from build123d import *

# Parameters (mm, degrees)
BOSS_EXTRUDE2_DEPTH = 27
BOSS_EXTRUDE3_DEPTH = 27
SKETCH2_W           = 35
SKETCH2_H           = 30
CUT_EXTRUDE1_DEPTH  = 5
FILLET1_R           = 1
SKETCH3_R           = 7.5
CUT_EXTRUDE2_DEPTH  = 1
FILLET2_R           = 1
FILLET3_R           = 1


with BuildPart() as part:
    # Sketch1 → Boss-Extrude2 (new body)
    with BuildSketch(Plane.XY):
        with BuildLine():
            Line((0, -6.138464618), (0, 24))
            Line((0, 24), (-18.5, 24))
            ThreePointArc((-18.5, 24), (-19.98907726, 20.440025069), (-23.569368605, 19.000481223))
            add(Edge.make_bspline(
                [(-38.977266034, 10), (-31.868069792, 12.073515571), (-23.569368605, 19.000481223)],
                knots=[0, 0, 0, 1, 1, 1], degree=2))
            add(Edge.make_bspline(
                [(-42.5, 0), (-60.990919768, 5.63165305), (-38.977266034, 10)],
                knots=[0, 0, 0, 1, 1, 1], degree=2))
            add(Edge.make_bspline(
                [(0, -6.138464618), (-21.18379083, -6.119278693), (-42.5, 0)],
                knots=[0.501567662, 0.501567662, 0.501567662, 1, 1, 1], degree=2))
        make_face()
    extrude(amount=BOSS_EXTRUDE2_DEPTH)

    # Sketch1_4 → Boss-Extrude3 (add)
    with BuildSketch(Plane.XY):
        with BuildLine():
            Line((18.5, 24), (0, 24))
            Line((0, 24), (0, -6.138464618))
            add(Edge.make_bspline(
                [(42.5, 0), (21.317044751, -6.157771231), (0, -6.138464618)],
                knots=[0, 0, 0, 0.501567662, 0.501567662, 0.501567662], degree=2))
            add(Edge.make_bspline(
                [(42.5, 0), (60.990919768, 5.63165305), (38.977266034, 10)],
                knots=[0, 0, 0, 1, 1, 1], degree=2))
            add(Edge.make_bspline(
                [(38.977266034, 10), (31.868069792, 12.073515571), (23.569368605, 19.000481223)],
                knots=[0, 0, 0, 1, 1, 1], degree=2))
            ThreePointArc((23.569368605, 19.000481223), (19.98907726, 20.440025069), (18.5, 24))
        make_face()
    extrude(amount=BOSS_EXTRUDE3_DEPTH)

    # Sketch2 → Cut-Extrude1 (cut)
    with BuildSketch(Plane(origin=(0, 0, 0), x_dir=(-1, 0, 0), z_dir=(0, 0, -1))):
        with Locations((0, 5)):
            Rectangle(SKETCH2_W, SKETCH2_H)
    extrude(amount=-CUT_EXTRUDE1_DEPTH, mode=Mode.SUBTRACT)

    # Fillet1
    fillet1_edges = [part.edges().sort_by_distance(p)[0] for p in [
        (17.5, 20, 2.5),
        (-17.5, 20, 2.5),
    ]]
    fillet(fillet1_edges, radius=FILLET1_R)

    # Sketch3 → Cut-Extrude2 (cut)
    with BuildSketch(Plane(origin=(0, 24, 0), x_dir=(1, 0, 0), z_dir=(0, 1, 0))):
        with Locations(Location((0, -13.5, 0), (0, 0, 270))):
            Circle(SKETCH3_R)
    extrude(amount=-CUT_EXTRUDE2_DEPTH, mode=Mode.SUBTRACT)

    # Fillet2
    fillet2_edges = [part.edges().sort_by_distance(p)[0] for p in [
        (-18.5, 24, 13.5),
    ]]
    fillet(fillet2_edges, radius=FILLET2_R)

    # Fillet3
    fillet3_edges = [part.edges().sort_by_distance(p)[0] for p in [
        (18.5, 24, 13.5),
    ]]
    fillet(fillet3_edges, radius=FILLET3_R)


solid = part.part
Verification items for the finished model (mm, model axes). A direction names the side the tool comes from. Round coordinates to 2 decimals unless told otherwise and drop trailing zeros. Write each loop counter-clockwise with the first axis right and the second up, starting at its lowest first coordinate (ties: lowest second). Pieces come first, ordered by that corner, then holes.
(1) Material ranges on line 1 (X direction, y = 4, z = 1.5); line 2 (X direction, y = 23.2, z = 13.5); line 3 (Z direction, x = 7.5, y = 8), recorded low to high.
Returned:
line 1: x = -50.64 to -17.5, 17.5 to 50.64
line 2: x = -18.56 to -7.5, 7.5 to 18.56
line 3: z = 5 to 27
(2) Access from +Z, -Z, +X, -X, +Y, -Y to the whole of each face (thin tool, end or side, straight path). Record for faces 1 (the cylindrical face through (6.324, 23.507, 17.532)), 2 (the flat face through (-1, 9, 27)), 3 (the flat face through (0, 7, 5)).
Returned:
face 1: +Y
face 2: +Z, +X, -X, +Y, -Y
face 3: -Z, -Y
(3) Mould release check, pull along X, two halves, no side actions. Record for faces 4 (the flat face through (4.2, 20.3, 0)), 5 (the flat face through (17.5, 7, 2)): pulls with the +X half, pulls with the -X half, needs draft (parallel to the pull), parting line crosses it, or undercut.
Returned:
face 4: needs draft
face 5: undercut
(4) Section check A-A (y = 21). Enter the section's corners in (x, z).
Returned:
outline: (-19.5, 0) - (19.5, 0) - (19.5, 27) - (-19.5, 27) - close
(5) Depth check by flat-ended pin: pin 1 Ø2.5 at (x, z) = (-1, 2.5) entering from -Y; pin 2 Ø5 at (x, z) = (-10.5, 13) entering from -Y; pin 3 Ø12 at (x, z) = (0, 13.5) entering from +Y. Enter the tip coordinate at first touch or a pass-through.
Returned:
pin 1: stops at y = 20
pin 2: stops at y = -5.91
pin 3: stops at y = 23
